Model file for the job. Use its own axes, mm. A direction names the side the tool comes from. Give positions to 0.01 mm unless a question says otherwise; leave off trailing zeros. Loops run counter-clockwise (first coordinate to the right, second up) from the corner with the lowest first, then second, coordinate; pieces in that order, holes last. Notation, with made-up numbers: M -9.75,43.25 L 27.25,43.25 A26 cw 27.25,81.25 Z; hole C -3,-28.75 d1. An arc over 180 degrees is marked long. Answer in a Markdown table with one row per item.
```python
from build123d import *

# Parameters (mm, degrees)
F0_W     = 255.5983066559
F0_H     = 256.2570720911
F1_DEPTH = 254
F2_T     = -2.54
F4_DEPTH = 253.492


with BuildPart() as f1:
    # F0 (on Top) → F1 (new body)
    with BuildSketch(Plane.XY):
        with Locations((-22.7167755365, -10.7608214021)):
            Rectangle(F0_W, F0_H)
    extrude(amount=F1_DEPTH)

    # F2
    f2_openings = [f1.faces().sort_by_distance(p)[0] for p in [
        (-22.716776, -138.889357, 127),
    ]]
    offset(amount=F2_T, openings=f2_openings)

    # F3 (on face) → F4 (join)
    with BuildSketch(Plane.XZ.offset(-114.8277146435)):
        Polygon((102.5423777914, 119.3862035871), (102.5423777914, 127), (102.5423777914, 134.8422765732), (-147.9759288645, 134.8422765732), (-147.9759288645, 119.3862035871), align=None)
    extrude(amount=F4_DEPTH)


solid = f1.part
```
(1) Which spindle directions (+Z, -Z, +X, -X, +Y, -Y) get a long thin tool onto all of the face, cutting with end or side? Do faces 4 (the flat face through (-24, -10, 251.46)), 5 (the flat face through (105.082, -13, 125)). Say none if no direction does.
Established:
| item | result |
|---|---|
| face 4 | -Y |
| face 5 | +Z, -Z, +X, +Y, -Y |
(2) Wall check: L1, parallel to Z at x = 31, y = -64; L2, parallel to X at y = -105, z = 136.5; L3, parallel to Y at x = 41, z = 130.5. Give the ranges that are in metal, low to high.
Established:
| item | result |
|---|---|
| L1 | z = 0 to 2.54, 119.39 to 134.84, 251.46 to 254 |
| L2 | x = -150.52 to -147.98, 102.54 to 105.08 |
| L3 | y = -138.66 to 117.37 |
(3) Flat gauge pins, fed straight in: P1, Ø8, axis at x = -35.5, z = 139, coming from the -Y side; P2, Ø7.5, axis at x = -42, z = 128, coming from the -Y side. Where does each tip first touch, or does it go through?
Established:
| item | result |
|---|---|
| P1 | stops at y = 114.83 |
| P2 | stops at y = -138.66 |
(4) Saw through at C-C, the plane z = 185. Give the cut face in (x, y), and give its area (3 significant figures).
Established:
| item | result |
|---|---|
| outline | M -150.52,-138.89 L -147.98,-138.89 L -147.98,114.83 L 102.54,114.83 L 102.54,-138.89 L 105.08,-138.89 L 105.08,117.37 L -150.52,117.37 Z |
| area | 1,940 mm2 |
(5) Mould opens along Z. For faces 1 (the flat face through (-25, -9, 0)), 2 (the flat face through (-25, -9, 254)), 3 (the flat face through (-24, -10, 2.54)) say: pulls with the +Z half, pulls with the -Z half, needs draft (parallel to the pull), parting line crosses it, or undercut.
Established:
| item | result |
|---|---|
| face 1 | pulls with the -Z half |
| face 2 | pulls with the +Z half |
| face 3 | undercut |
(6) Saw through at A-A, the plane y = -34.5. Give the cut face in (x, z), and give its area (4 significant figures).
Established:
| item | result |
|---|---|
| outline | M -150.52,0 L 105.08,0 L 105.08,254 L -150.52,254 Z; hole M -147.98,2.54 L 102.54,2.54 L 102.54,119.39 L -147.98,119.39 Z; hole M -147.98,134.84 L 102.54,134.84 L 102.54,251.46 L -147.98,251.46 Z |
| area | 6,435 mm2 |
(7) Saw through at B-B, the plane x = -73.5. Give the cut face in (y, z), and give its area (3 significant figures).
Established:
| item | result |
|---|---|
| outline | M -138.89,0 L 117.37,0 L 117.37,254 L -138.89,254 L -138.89,251.46 L 114.83,251.46 L 114.83,134.84 L -138.66,134.84 L -138.66,119.39 L 114.83,119.39 L 114.83,2.54 L -138.89,2.54 Z |
| area | 5,850 mm2 |
